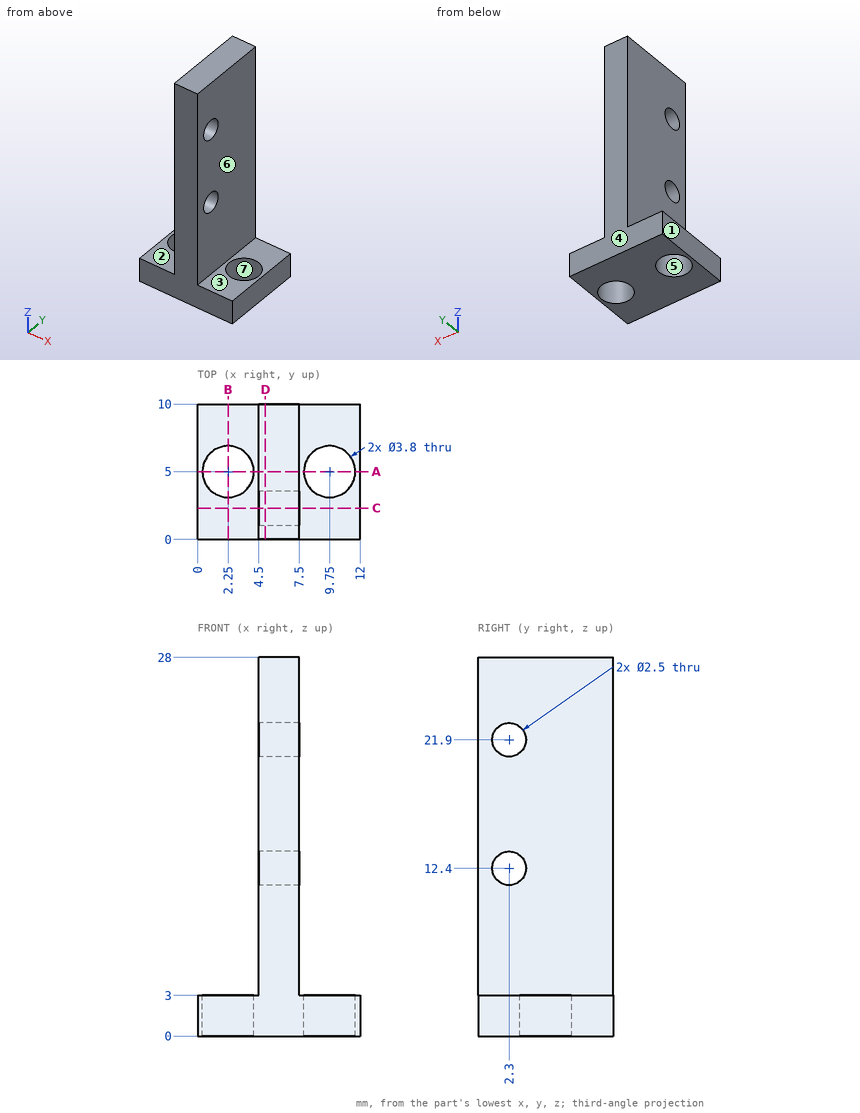
The figure shows three views and two pictorial views of one solid part (mm, origin at its lowest corner). Answer the questions. A direction names the side the tool comes from. Coordinates: 2 decimals unless noted, no trailing zeros. Loops run counter-clockwise (first coordinate to the right, second up) from the corner with the lowest first, then second, coordinate; pieces in that order, holes last.
1) Find section B-B on x = 2.25. Write down the section's boundary in (y, z).
2) Find section C-C on y = 2.3. Write down the section's boundary in (x, z), then the cut area to 3 significant figures.
3) Flat-ended cylindrical pins translate along their axes: pin 1 Ø1.5 at (y, z) = (8.5, 19.5) entering from +X; pin 2 Ø2 at (y, z) = (2.3, 12.4) entering from -X; pin 3 Ø5 at (y, z) = (7.5, 19) entering from -X; pin 4 Ø2.5 at (x, y) = (9, 5.5) entering from +Z. Find the tip coordinate at first contact, or state that the pin passes through.
4) Find section D-D on x = 5. Write down the section's boundary in (y, z).
5) A tool of negligible diameter and unlimited length cuts with its end or side. For the marked faces 1, 2 and 3, from which of +Z, -Z, +X, -X, +Y, -Y can it reach the whole face along a straight path? Write none if from no direction.
6) Determine the mould class of the marked faces 4, 5, 6 and 7 for opening direction X: pulls with the +X half, pulls with the -X half, needs draft (parallel to the pull), parting line crosses it, or undercut.
7) Find section A-A on y = 5. Write down the section's boundary in (x, z), then the cut area to 3 significant figures.
8) Find the intervals of material crossed by L1, parallel to Z at x = 5.6, y = 2.3; L2, parallel to X at y = 5, z = 0.7; L3, parallel to Y at x = 2.25, z = 2.3, in increasing order.
Values:
1. outline: (0, 0) - (3.1, 0) - (3.1, 3) - (0, 3) - close; (6.9, 0) - (10, 0) - (10, 3) - (6.9, 3) - close
2. outline: (0, 0) - (12, 0) - (12, 3) - (7.5, 3) - (7.5, 11.15) - (4.5, 11.15) - (4.5, 3) - (0, 3) - close; (4.5, 13.65) - (7.5, 13.65) - (7.5, 20.65) - (4.5, 20.65) - close; (4.5, 23.15) - (7.5, 23.15) - (7.5, 28) - (4.5, 28) - close
2. area: 96.0 mm2
3. pin 1: stops at x = 7.5
3. pin 2: passes through
3. pin 3: stops at x = 4.5
3. pin 4: stops at z = 3
4. outline: (0, 0) - (10, 0) - (10, 28) - (0, 28) - close; hole circle Ø2.5 at (2.3, 12.4); hole circle Ø2.5 at (2.3, 21.9)
5. face 1: +Z, -Z, -X, +Y, -Y
5. face 2: +Z, -X, +Y, -Y
5. face 3: +Z, +X, +Y, -Y
6. face 4: needs draft
6. face 5: undercut
6. face 6: pulls with the +X half
6. face 7: undercut
7. outline: (0, 0) - (0.35, 0) - (0.35, 3) - (0, 3) - close; (4.15, 0) - (7.85, 0) - (7.85, 3) - (7.5, 3) - (7.5, 28) - (4.5, 28) - (4.5, 3) - (4.15, 3) - close; (11.65, 0) - (12, 0) - (12, 3) - (11.65, 3) - close
7. area: 88.2 mm2
8. L1: z = 0 to 11.15, 13.65 to 20.65, 23.15 to 28
8. L2: x = 0 to 0.35, 4.15 to 7.85, 11.65 to 12
8. L3: y = 0 to 3.1, 6.9 to 10
